Could you check a few things on this drawing? It's one solid part, dimensions in mm from its lowest x, y, z. Coordinates: 2 decimals unless noted, no trailing zeros. Write each loop counter-clockwise with the first axis right and the second up, starting at its lowest first coordinate (ties: lowest second). Pieces come first, ordered by that corner, then holes.
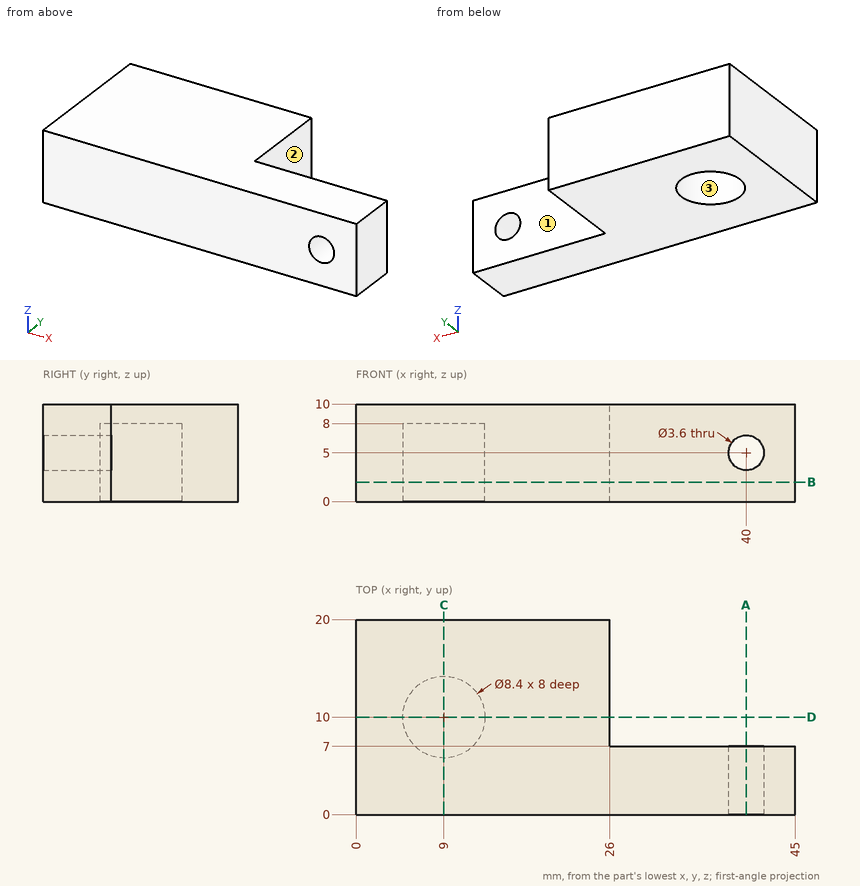
1) Imagine slicing it at B-B on z = 2. Please give me the cut outline in (x, y).
Values follow:
outline: (0, 0) - (45, 0) - (45, 7) - (26, 7) - (26, 20) - (0, 20) - close; hole circle Ø8.4 at (9, 10)
2) I need wall thicknesses on probe 1 along Y at (x, z) = (9, 5); probe 2 along X at (y, z) = (2, 5); probe 3 along X at (y, z) = (10, 4.25). Which ranges of each line are inside material? Lowest first, please.
Values follow:
probe 1: y = 0 to 5.8, 14.2 to 20
probe 2: x = 0 to 38.2, 41.8 to 45
probe 3: x = 0 to 4.8, 13.2 to 26
3) Imagine slicing it at D-D on y = 10. Please give me the cut outline in (x, z).
Values follow:
outline: (0, 0) - (4.8, 0) - (4.8, 8) - (13.2, 8) - (13.2, 0) - (26, 0) - (26, 10) - (0, 10) - close
4) Imagine slicing it at A-A on x = 40. Please give me the cut outline in (y, z).
Values follow:
outline: (0, 0) - (7, 0) - (7, 3.2) - (0, 3.2) - close; (0, 6.8) - (7, 6.8) - (7, 10) - (0, 10) - close
5) Will these pins go through, and if not, where does the flat tip stop? pin 1 (3 mm diameter, centred on y = 11, z = 3.5, fed in from +X); pin 2 (5 mm diameter, centred on x = 32.5, z = 5, fed in from +Y).
Values follow:
pin 1: stops at x = 26
pin 2: stops at y = 7
6) Imagine slicing it at C-C on x = 9. Please give me the cut outline in (y, z), then the cut area to 3 significant figures.
Values follow:
outline: (0, 0) - (5.8, 0) - (5.8, 8) - (14.2, 8) - (14.2, 0) - (20, 0) - (20, 10) - (0, 10) - close
area: 133 mm2
7) We'd pull the mould along Y, two halves only. Please class the marked faces 1, 2 and 3: pulls with the +Y half, pulls with the -Y half, needs draft (parallel to the pull), parting line crosses it, or undercut.
Values follow:
face 1: pulls with the +Y half
face 2: needs draft
face 3: undercut
